from build123d import *

# Parameters (mm, degrees)
PAD_DEPTH       = 55
SKETCH001_W     = 49
SKETCH001_H     = 60.9
POCKET_DEPTH    = 500
POCKET001_DEPTH = 500


with BuildPart() as part:
    # Sketch → Pad (new body)
    with BuildSketch(Plane.YZ):
        with BuildLine():
            ThreePointArc((28.980657, 15.850683), (42.584206, 34.802551), (21.20392, 44.135996))
            Line((-52.001908, 0), (21.20392, 44.135996))
            ThreePointArc((-52.001908, 0), (-53.920439, -24.881725), (-30.209248, -17.099671))
            ThreePointArc((28.980657, 15.850683), (-4.124344, 5.680733), (-30.209248, -17.099671))
        make_face()
    extrude(amount=PAD_DEPTH)

    # Sketch001 → Pocket (cut)
    with BuildSketch(Plane(origin=(27.5, 23, -50), x_dir=(1, 0, 0), z_dir=(0, 0, 1))):
        Rectangle(SKETCH001_W, SKETCH001_H)
    extrude(amount=POCKET_DEPTH, mode=Mode.SUBTRACT)

    # Sketch002 → Pocket001 (cut)
    with BuildSketch(Plane(origin=(27.5, -35, -50), x_dir=(1, 0, 0), z_dir=(0, 0, 1))):
        with BuildLine():
            Line((-49.999941, -8.209968), (-49.999941, -38.209968))
            Line((-49.999941, -38.209968), (-15, -38.209968))
            Line((-15, -38.209968), (-15, -7.838993))
            ThreePointArc((-15, -7.838993), (-25.381364, 16.670931), (-49.999941, 26.791938))
            Line((-49.999941, 26.791938), (-49.999941, -8.209968))
        make_face()
        with BuildLine():
            Line((15, -7.838993), (15, -38.220366))
            Line((15, -38.220366), (49.997922, -38.220366))
            Line((49.997922, -38.220366), (49.997922, -8.220366))
            Line((49.99995, 26.779634), (49.997922, -8.220366))
            ThreePointArc((49.99995, 26.779634), (25.385111, 16.663555), (15, -7.838993))
        make_face()
    extrude(amount=POCKET001_DEPTH, mode=Mode.SUBTRACT)


solid = part.part
CAD build for the part. Positions are in the model's coordinates, mm. A direction names the side the tool comes from. Give positions to 0.01 mm unless a question says otherwise; leave off trailing zeros. Order: outer loops, then holes, each group sorted by start corner. A loop starts at its lowest first (then second) coordinate and runs counter-clockwise, first axis right, second up. Notation, with made-up numbers: (-13.5, 46.5) -> (9.5, 46.5) arc R18 ccw to (9.5, 70.5) -> close; hole circle Ø4 at (78, 53.25). An arc over 180 degrees is marked (long way). Return JSON: item names as keys, results as strings.
Q1. Drill centre lines: line 1 (X direction, y = 20.5, z = 31.5); line 2 (X direction, y = -44.5, z = -25); line 3 (Y direction, x = 30.5, z = 15). Where is each one in solid material? Low to high.
Working result:
{"line 1": "0 to 3, 52 to 55", "line 2": "12.5 to 42.5", "line 3": "-27.12 to -7.45"}
Q2. Saw through at C-C (x = 16). Write the cut outline in (y, z).
Working result:
{"outline": "(-52, 0) arc R15 ccw (long way) to (-30.21, -17.1) arc R83.1 cw to (-7.45, 3.73) -> (-7.45, 26.86) -> close"}
Q3. Flat gauge pins, fed straight in: pin 1 (8 mm diameter, centred on x = 12.5, z = -20.5, fed in from -Y); pin 2 (7 mm diameter, centred on x = 30, z = 16, fed in from +Y); pin 3 (8.5 mm diameter, centred on y = -48.5, z = -18, fed in from -X); pin 4 (8 mm diameter, centred on y = 20.5, z = 28.5, fed in from -X). Where does each tip first touch, or does it go through?
Working result:
{"pin 1": "y = -59.27", "pin 2": "y = -7.45", "pin 3": "x = 12.5", "pin 4": "x = 0"}
Q4. Saw through at A-A (y = 22.5). Write the cut outline in (x, z).
Working result:
{"outline": "(0, 15.02) -> (3, 15.02) -> (3, 44.73) -> (0, 44.73) -> close; (52, 15.02) -> (55, 15.02) -> (55, 44.73) -> (52, 44.73) -> close"}
Q5. Mould opens along X. For faces 1 (the face through (52, 17, 24)), 2 (the face through (42.5, -49, -12)), 3 (the face through (27.115, -24.045, 16.855)) say: pulls with the +X half, pulls with the -X half, needs draft (parallel to the pull), parting line crosses it, or undercut.
Working result:
{"face 1": "undercut", "face 2": "pulls with the +X half", "face 3": "needs draft"}
Q6. Saw through at B-B (z = 40.5). Write the cut outline in (x, y).
Working result:
{"outline": "(0, 15.17) -> (3, 15.17) -> (3, 39.58) -> (0, 39.58) -> close; (52, 15.17) -> (55, 15.17) -> (55, 39.58) -> (52, 39.58) -> close"}
Q7. Saw through at D-D (z = -13.5). Write the cut outline in (x, y) (3 decimals).
Working result:
{"outline": "(8.704, -27.354) arc R35.002 cw to (12.5, -42.839) -> (12.5, -59.655) -> (42.5, -59.655) -> (42.5, -42.839) arc R35 cw to (46.301, -27.354) -> close"}
Q8. Which spindle directions (+Z, -Z, +X, -X, +Y, -Y) get a long thin tool onto all of the face, cutting with end or side? Do faces 4 (the face through (12.5, -49, -12)), 5 (the face through (27, -7.45, 15)), 6 (the face through (45.949, -28.066, -3.601)). Say none if no direction does.
Working result:
{"face 4": "+Z, -Z, -X, -Y", "face 5": "+Z, -Z, +Y", "face 6": "+Z, -Z, +X, -Y"}
